from build123d import *

# Parameters (mm, degrees)
F0_R     = 9.95
F1_DEPTH = 6


# Not quite as in the source:
# - a feature names something its author has since deleted; it is built from what else it names


with BuildPart() as f1:
    # F0 (on Top) → F1 (new body)
    with BuildSketch(Plane.XY):
        with BuildLine():
            ThreePointArc((8.2915619759, 12.5), (0, 40), (-8.2915619759, 12.5))
            ThreePointArc((-8.2915619759, 12.5), (-10.9307033082, 10.2722794544), (-12.9903810568, 7.5))
            ThreePointArc((-12.9903810568, 7.5), (-14.3614066163, 4.3301270189), (-14.9710985352, 0.9307033082))
            ThreePointArc((-14.9710985352, 0.9307033082), (-34.6410161514, -20), (-6.6795365594, -13.4307033082))
            ThreePointArc((-6.6795365594, -13.4307033082), (-3.4307033082, -14.6024064733), (0, -15))
            ThreePointArc((0, -15), (3.4307033082, -14.6024064733), (6.6795365594, -13.4307033082))
            ThreePointArc((6.6795365594, -13.4307033082), (34.6410161514, -20), (14.9710985352, 0.9307033082))
            ThreePointArc((14.9710985352, 0.9307033082), (14.3614066163, 4.3301270189), (12.9903810568, 7.5))
            ThreePointArc((12.9903810568, 7.5), (10.9307033082, 10.2722794544), (8.2915619759, 12.5))
        make_face()
        with Locations((-21.6506350946, -12.5)):
            Circle(F0_R, mode=Mode.SUBTRACT)
        with Locations((21.6506350946, -12.5)):
            Circle(F0_R, mode=Mode.SUBTRACT)
        with BuildLine():
            ThreePointArc((0, 11), (5.5, 9.5262794416), (9.5262794416, 5.5))
            ThreePointArc((9.5262794416, 5.5), (9.5262794416, -5.5), (0, -11))
            ThreePointArc((0, -11), (-9.5262794416, -5.5), (-9.5262794416, 5.5))
            ThreePointArc((-9.5262794416, 5.5), (-5.5, 9.5262794416), (0, 11))
        make_face(mode=Mode.SUBTRACT)
        with BuildLine():
            ThreePointArc((9.95, 25), (7.0357124728, 17.9642875272), (0, 15.05))
            ThreePointArc((0, 15.05), (-7.0357124728, 32.0357124728), (9.95, 25))
        make_face(mode=Mode.SUBTRACT)
    extrude(amount=F1_DEPTH)


solid = f1.part
Input: part model. Units: mm. Frame: model coordinates. Round coordinates to 2 decimals unless told otherwise and drop trailing zeros. Write each loop counter-clockwise with the first axis right and the second up, starting at its lowest first coordinate (ties: lowest second). Pieces come first, ordered by that corner, then holes.
1) Cut plane D-D (y = 20.5). Return the cut outline in (x, z), then the cut area to 3 significant figures.
2) Contact query for a flat-ended pin moving along its axis: P1, Ø5, axis at x = 19, y = 2.5, coming from the +Z side. Output: stop coordinate, or through.
3) Cut plane C-C (y = -4). Return the cut outline in (x, z), then the cut area to 3 significant figures.
4) Cut plane A-A (z = 3.1). Return the cut outline in (x, y).
5) Ray query, L1, parallel to Y at x = 3.5, z = 5.7; L2, parallel to Y at x = 13, z = 5.05; L3, parallel to Y at x = 23, z = 2.6. Return the intervals inside material, ascending.
6) Draft query along Y for faces 1 (the flat face through (3, 11, 6)), 2 (the cylindrical face through (-23.808, -22.213, 2.958)). Return one class per face: pulls with the +Y half, pulls with the -Y half, needs draft (parallel to the pull), parting line crosses it, or undercut.
7) Cut plane B-B (y = -12.5). Return the cut outline in (x, z).
Geometry says:
1. outline: (-14.31, 0) - (-8.87, 0) - (-8.87, 6) - (-14.31, 6) - close; (8.87, 0) - (14.31, 0) - (14.31, 6) - (8.87, 6) - close
1. area: 65.2 mm2
2. P1: stops at z = 6
3. outline: (-34.01, 0) - (-26.82, 0) - (-26.82, 6) - (-34.01, 6) - close; (-16.48, 0) - (-10.25, 0) - (-10.25, 6) - (-16.48, 6) - close; (10.25, 0) - (16.48, 0) - (16.48, 6) - (10.25, 6) - close; (26.82, 0) - (34.01, 0) - (34.01, 6) - (26.82, 6) - close
3. area: 161 mm2
4. outline: (-14.97, 0.93) arc R15 ccw (long way) to (-6.68, -13.43) arc R15 ccw to (6.68, -13.43) arc R15 ccw (long way) to (14.97, 0.93) arc R15 ccw to (8.29, 12.5) arc R15 ccw (long way) to (-8.29, 12.5) arc R15 ccw to start; hole circle Ø19.9 at (-21.65, -12.5); hole circle Ø22 at (0, 0); hole circle Ø19.9 at (0, 25); hole circle Ø19.9 at (21.65, -12.5)
5. L1: y = -14.59 to -10.43, 10.43 to 15.69, 34.31 to 39.59
5. L2: y = -24.75 to -17.42, -7.58 to 7.48, 17.52 to 32.48
5. L3: y = -27.44 to -22.36, -2.64 to 2.44
6. face 1: needs draft
6. face 2: undercut
7. outline: (-36.65, 0) - (-31.6, 0) - (-31.6, 6) - (-36.65, 6) - close; (-11.7, 0) - (11.7, 0) - (11.7, 6) - (-11.7, 6) - close; (31.6, 0) - (36.65, 0) - (36.65, 6) - (31.6, 6) - close
